Could you check a few things on this drawing? It's one solid part, dimensions in mm from its lowest x, y, z. Give positions to 0.01 mm unless a question says otherwise; leave off trailing zeros. Loops run counter-clockwise (first coordinate to the right, second up) from the corner with the lowest first, then second, coordinate; pieces in that order, holes last.
1. Imagine slicing it at A-A (x = 88.25). List the corners of the cut face in (y, z) for me, plus the area to 3 significant figures.
2. I need wall thicknesses on line 1 along X through (y, z) = (2.3, 19); line 2 along Z through (x, y) = (8, 3.2); line 3 along Z through (x, y) = (89.5, 2.45). Which ranges of each line are inside material? Lowest first, please.
3. Imagine slicing it at B-B (y = 1.55). List the corners of the cut face in (x, z) for me.
4. Imagine slicing it at C-C (z = 26). List the corners of the cut face in (x, y) for me.
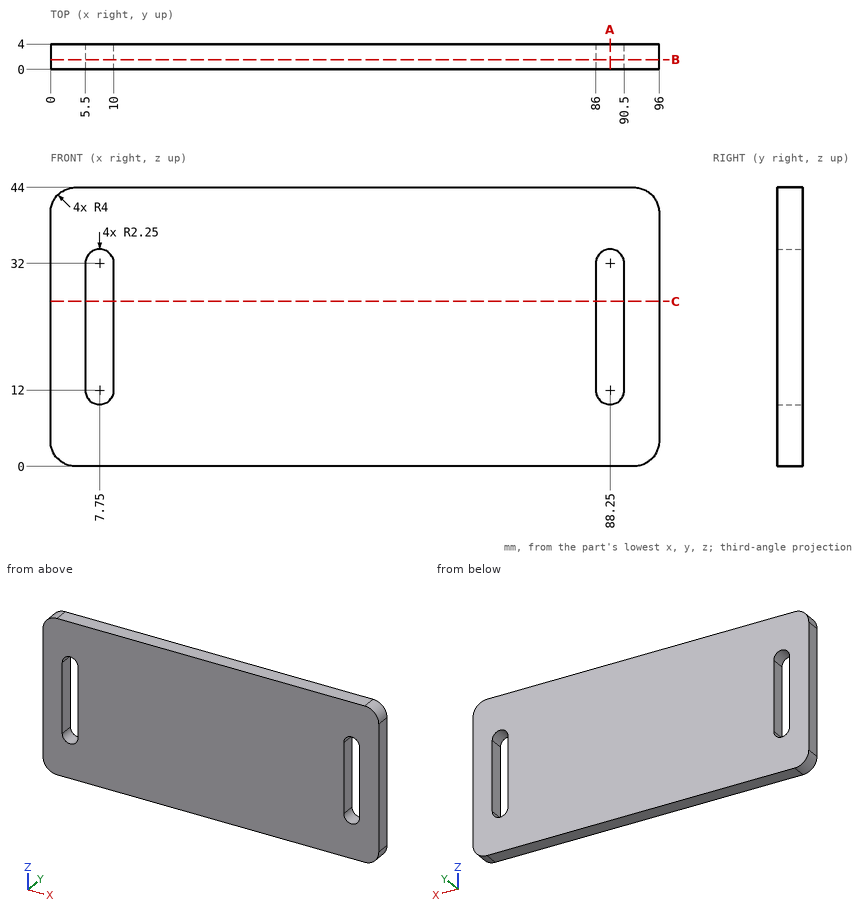
Derived:
1. outline: (0, 0) - (4, 0) - (4, 9.75) - (0, 9.75) - close; (0, 34.25) - (4, 34.25) - (4, 44) - (0, 44) - close
1. area: 78.0 mm2
2. line 1: x = 0 to 5.5, 10 to 86, 90.5 to 96
2. line 2: z = 0 to 9.76, 34.24 to 44
2. line 3: z = 0 to 10.13, 33.87 to 44
3. outline: (0, 4) arc R4 ccw to (4, 0) - (92, 0) arc R4 ccw to (96, 4) - (96, 40) arc R4 ccw to (92, 44) - (4, 44) arc R4 ccw to (0, 40) - close; hole (5.5, 12) arc R2.25 ccw to (10, 12) - (10, 32) arc R2.25 ccw to (5.5, 32) - close; hole (86, 12) arc R2.25 ccw to (90.5, 12) - (90.5, 32) arc R2.25 ccw to (86, 32) - close
4. outline: (0, 0) - (5.5, 0) - (5.5, 4) - (0, 4) - close; (10, 0) - (86, 0) - (86, 4) - (10, 4) - close; (90.5, 0) - (96, 0) - (96, 4) - (90.5, 4) - close
